Build history of the part. All positions in model axes, mm. A direction names the side the tool comes from. Give positions to 0.01 mm unless a question says otherwise; leave off trailing zeros. Order: outer loops, then holes, each group sorted by start corner. A loop starts at its lowest first (then second) coordinate and runs counter-clockwise, first axis right, second up. Notation, with made-up numbers: (-12, 63) - (12, 63) arc R10 cw to (12, 82) - close; hole circle Ø9 at (31, 12.25). An arc over 180 degrees is marked (long way). One line per item, written item: value.
```python
from build123d import *

# Parameters (mm, degrees)
SKETCH_1_R          = 3
EXTRUDE_1_DEPTH     = 16
CUT_EXTRUDE_1_REACH = 84.476
SKETCH_2_R          = 3
CUT_EXTRUDE_2_REACH = 84.476
CUT_EXTRUDE_3_DEPTH = 30
SKETCH_5_R          = 3
CUT_EXTRUDE_4_DEPTH = 78.517739905
EXTRUDE_START       = 1
SKETCH_6_R          = 6
SKETCH_6_R_2        = 3
EXTRUDE_2_DEPTH     = 1
FILLET_1_R          = 7
FILLET_START        = -27
FILLET_3_DEPTH      = 69
FILLET_START_2      = -3.5
FILLET_3_2_DEPTH    = 30


with BuildPart() as part:
    # 草图1 → 凸台-拉伸1 (new body)
    with BuildSketch(Plane(origin=(0, 0, 0), x_dir=(1, 0, 0), z_dir=(0, 1, 0))):
        Polygon((-3.5, 64), (26.5, 64), (26.5, 29), (43, 29), (43, -10), (31.5, -10), (21.5, -25), (21.5, -48), (1.5, -48), (1.5, -25), (-8.5, -10), (-28, -10), (-28, 29), (-3.5, 29), align=None)
        with Locations(Location((-20, 0, 0), (0, 0, 270))):
            Circle(SKETCH_1_R, mode=Mode.SUBTRACT)
        with Locations(Location((35, 14, 0), (0, 0, 270))):
            Circle(SKETCH_1_R, mode=Mode.SUBTRACT)
        with BuildLine():
            Line((6.140864253, -6.579497414), (21.140864253, 7.420502586))
            ThreePointArc((21.140864253, 7.420502586), (21.579497414, 20.140864253), (8.859135747, 20.579497414))
            Line((8.859135747, 20.579497414), (-6.140864253, 6.579497414))
            ThreePointArc((-6.140864253, 6.579497414), (-6.579497414, -6.140864253), (6.140864253, -6.579497414))
        make_face(mode=Mode.SUBTRACT)
    extrude(amount=EXTRUDE_1_DEPTH)

    # 草图2 → 切除-拉伸1 (cut, up to next)
    with BuildSketch(Plane(origin=(21.5, 0, 0), x_dir=(0, 0, -1), z_dir=(1, 0, 0)), mode=Mode.PRIVATE) as cut_extrude_1_sk1:
        with Locations((-40, 8)):
            Circle(SKETCH_2_R)
    cut_extrude_1_tool1 = extrude(cut_extrude_1_sk1.sketch, amount=-CUT_EXTRUDE_1_REACH, mode=Mode.PRIVATE) & part.part
    add(cut_extrude_1_tool1.solids().sort_by_distance((21.5, 8, 40))[0], mode=Mode.SUBTRACT)

    # 草图3 → 切除-拉伸2 (cut, up to next)
    with BuildSketch(Plane(origin=(21.5, 0, 0), x_dir=(0, 0, -1), z_dir=(1, 0, 0)), mode=Mode.PRIVATE) as cut_extrude_2_sk1:
        with BuildLine():
            ThreePointArc((-48, 8), (-45.656854249, 13.656854249), (-40, 16))
            Line((-40, 16), (-48, 16))
            Line((-48, 16), (-48, 8))
        make_face()
    cut_extrude_2_tool1 = extrude(cut_extrude_2_sk1.sketch, amount=-CUT_EXTRUDE_2_REACH, mode=Mode.PRIVATE) & part.part
    # 草图3 → 切除-拉伸2 (cut, up to next)
    with BuildSketch(Plane(origin=(21.5, 0, 0), x_dir=(0, 0, -1), z_dir=(1, 0, 0)), mode=Mode.PRIVATE) as cut_extrude_2_sk2:
        with BuildLine():
            Line((-48, 0), (-40, 0))
            ThreePointArc((-40, 0), (-45.656854249, 2.343145751), (-48, 8))
            Line((-48, 8), (-48, 0))
        make_face()
    cut_extrude_2_tool2 = extrude(cut_extrude_2_sk2.sketch, amount=-CUT_EXTRUDE_2_REACH, mode=Mode.PRIVATE) & part.part
    add(cut_extrude_2_tool1.solids().sort_by_distance((21.5, 14.213056, 46.213056))[0], mode=Mode.SUBTRACT)
    add(cut_extrude_2_tool2.solids().sort_by_distance((21.5, 1.786944, 46.213056))[0], mode=Mode.SUBTRACT)

    # 草图4 → 切除-拉伸3 (cut)
    with BuildSketch(Plane(origin=(26.5, 0, 0), x_dir=(0, 0, -1), z_dir=(1, 0, 0))):
        Polygon((29, 16), (64, 16), (64, 8), (44, 8), align=None)
    extrude(amount=-CUT_EXTRUDE_3_DEPTH, mode=Mode.SUBTRACT)

    # 草图5 → 切除-拉伸4 (cut, through all)
    with BuildSketch(Plane(origin=(0, 8, 0), x_dir=(1, 0, 0), z_dir=(0, 1, 0))):
        with Locations(Location((11.5, 54, 0), (0, 0, 270))):
            Circle(SKETCH_5_R)
    extrude(amount=-CUT_EXTRUDE_4_DEPTH, mode=Mode.SUBTRACT)

    # 草图6 → 凸台-拉伸2 (add)
    with BuildSketch(Plane(origin=(0, 8, 0), x_dir=(1, 0, 0), z_dir=(0, 1, 0)).offset(EXTRUDE_START)):
        with Locations(Location((11.5, 54, 0), (0, 0, 90))):
            Circle(SKETCH_6_R)
        with Locations(Location((11.5, 54, 0), (0, 0, 270))):
            Circle(SKETCH_6_R_2, mode=Mode.SUBTRACT)
    extrude(amount=-EXTRUDE_2_DEPTH)

    # 圆角1
    fillet_1_edges = [part.edges().sort_by_distance(p)[0] for p in [
        (1.5, 8, 25),
        (-8.5, 8, 10),
        (-28, 8, 10),
        (-28, 8, -29),
        (-3.5, 8, -29),
        (26.5, 8, -29),
        (43, 8, -29),
        (43, 8, 10),
        (31.5, 8, 10),
        (21.5, 8, 25),
    ]]
    fillet(fillet_1_edges, radius=FILLET_1_R)

    # 圆角3: read off the stored shape, not the designer's step
    # 圆角3 outline → 圆角3 (cut)
    with BuildSketch(Plane.YZ.offset(FILLET_START)):
        with BuildLine():
            Line((14.823529412, -31.205882353), (16, -29))
            Line((16, -29), (16, -26.5))
            ThreePointArc((16, -26.5), (15.701425001, -28.92535625), (14.823529412, -31.205882353))
        make_face()
    extrude(amount=FILLET_3_DEPTH, mode=Mode.SUBTRACT)

    # Fillet 3 2 outline → Fillet 3 2 (add)
    with BuildSketch(Plane.YZ.offset(FILLET_START_2)):
        with BuildLine():
            Line((8, -44), (8, -46.5))
            ThreePointArc((8, -46.5), (8.298574999, -44.07464375), (9.176470588, -41.794117647))
            Line((9.176470588, -41.794117647), (8, -44))
        make_face()
    extrude(amount=FILLET_3_2_DEPTH)


solid = part.part
```
(1) Slice it at D-D, the plane z = 5. Give the cut face in (x, y).
Completed:
outline: (-27.71, 0) - (-7.48, 0) - (-7.48, 16) - (-27.71, 16) - close; (7.83, 0) - (42.71, 0) - (42.71, 16) - (7.83, 16) - close
(2) Slice it at B-B, the plane x = 11.5. Give the cut face in (y, z).
Completed:
outline: (0, -64) - (8, -64) - (8, -60) - (9, -60) - (9, -57) - (0, -57) - close; (0, -51) - (9, -51) - (9, -48) - (8, -48) - (8, -46.5) arc R10 cw to (9.18, -41.79) - (14.82, -31.21) arc R10 ccw to (16, -26.5) - (16, -22.29) - (0, -22.29) - close; (0, 1.58) - (16, 1.58) - (16, 40) arc R8 ccw to (0, 40) - close; hole circle Ø6 at (8, 40)
(3) Drill centre lines: line 1 (Z direction, x = 19, y = 9); line 2 (X direction, y = 7, z = -54); line 3 (Z direction, x = 17, y = 9.5). Where is each one in solid material? Low to high.
Completed:
line 1: -42.14 to -22.06, -5.42 to 37.17, 42.83 to 47.94
line 2: -3.5 to 8.5, 14.5 to 26.5
line 3: -41.19 to -22.77, -3.56 to 37.4, 42.6 to 47.86
(4) Pull direction X, two halves, no side cores. Call faces 1 (the face through (11.6, 4.6, -57)), 2 (the face through (1.21, 8.11, 25.12)), 3 (the face through (12, 8, 43)): +X half, -X half, draft (parallel to the pull), parting line (faces both ways), or undercut.
Completed:
face 1: undercut
face 2: -X half
face 3: draft
(5) 3-axis set-ups, long thin cutter, end or side, ignore diameter. For faces 4 (the face through (21.5, 8, 35)), 5 (the face through (26.5, 5, -50)), 6 (the face through (-3.5, 5, -50)): which of +Z, -Z, +X, -X, +Y, -Y reach the whole face in a straight line?
Completed:
face 4: +Z, +X, +Y, -Y
face 5: -Z, +X, +Y, -Y
face 6: -Z, -X, +Y, -Y
(6) Slice it at A-A, the plane z = -54. Give the cut face in (x, y).
Completed:
outline: (-3.5, 0) - (8.5, 0) - (8.5, 9) - (5.5, 9) - (5.5, 8) - (-3.5, 8) - close; (14.5, 0) - (26.5, 0) - (26.5, 8) - (17.5, 8) - (17.5, 9) - (14.5, 9) - close
(7) Slice it at C-C, the plane z = -14. Give the cut face in (x, y), and give its area (3 significant figures).
Completed:
outline: (-28, 0) - (1.81, 0) - (1.81, 16) - (-28, 16) - close; (24, 0) - (32, 0) - (32, 16) - (24, 16) - close; (38, 0) - (43, 0) - (43, 16) - (38, 16) - close
area: 685 mm²
(8) Pin check, flat tips, straight feed: P1, Ø6, axis at y = 5.5, z = -49, coming from the +X side; P2, Ø1.5, axis at x = 12.5, z = -51.5, coming from the +Y side; P3, Ø8, axis at y = 4, z = -39, coming from the -X side. Stop position of each tip, or through.
Completed:
P1: x = 26.5
P2: y = 9
P3: x = -3.57
